The listing builds one solid part. Answer for the finished solid, in the listing's coordinates (mm). A direction names the side the tool comes from. Give positions to 0.01 mm unless a question says otherwise; leave off trailing zeros. Order: outer loops, then holes, each group sorted by start corner. A loop starts at its lowest first (then second) coordinate and runs counter-clockwise, first axis right, second up. Notation, with made-up numbers: (36.5, 51.25) - (61.5, 51.25) arc R3 ccw to (61.5, 55.25) - close; hole circle Ø5 at (50, 63). An arc over 180 degrees is marked (long way). Use CSV: the item, a comma, the result in double quotes.
```python
from build123d import *

# Parameters (mm, degrees)
SKETCH_1_W          = 80
SKETCH_1_H          = 40
EXTRUDE_1_DEPTH     = 9
SKETCH_2_R          = 2.25
CUT_EXTRUDE_1_DEPTH = 46.617978912
SKETCH_3_R          = 2.25
CUT_EXTRUDE_2_DEPTH = 9
SKETCH_4_R          = 4
CUT_EXTRUDE_3_DEPTH = 4.5
SKETCH_6_R          = 4
CUT_EXTRUDE_5_DEPTH = 4.5


with BuildPart() as part:
    # 草图1 → 凸台-拉伸1 (new body)
    with BuildSketch(Plane.XY):
        Rectangle(SKETCH_1_W, SKETCH_1_H)
    extrude(amount=EXTRUDE_1_DEPTH)

    # 草图2 → 切除-拉伸1 (cut, through all)
    with BuildSketch(Plane(origin=(0, 0, 0), x_dir=(-1, 0, 0), z_dir=(0, 0, -1))):
        with Locations((30, 10)):
            Circle(SKETCH_2_R)
        with Locations((30, -10)):
            Circle(SKETCH_2_R)
    cut_extrude_1 = extrude(amount=-CUT_EXTRUDE_1_DEPTH, mode=Mode.SUBTRACT)

    # 镜向1: 切除-拉伸1 across plane
    add(cut_extrude_1.mirror(Plane(origin=(0, 0, 0), x_dir=(0, 0, 1), z_dir=(1, 0, 0))), mode=Mode.SUBTRACT)

    # 草图3 → 切除-拉伸2 (cut)
    with BuildSketch(Plane(origin=(0, 0, 0), x_dir=(-1, 0, 0), z_dir=(0, 0, -1))):
        with Locations((12.5, -12.5)):
            Circle(SKETCH_3_R)
        with Locations((12.5, 12.5)):
            Circle(SKETCH_3_R)
    cut_extrude_2 = extrude(amount=-CUT_EXTRUDE_2_DEPTH, mode=Mode.SUBTRACT)

    # 镜向2: 切除-拉伸2 across plane
    add(cut_extrude_2.mirror(Plane(origin=(0, 0, 0), x_dir=(0, 0, 1), z_dir=(1, 0, 0))), mode=Mode.SUBTRACT)

    # 草图4 → 切除-拉伸3 (cut)
    with BuildSketch(Plane(origin=(0, 0, 0), x_dir=(-1, 0, 0), z_dir=(0, 0, -1))):
        with Locations((12.5, 12.5)):
            Circle(SKETCH_4_R)
        with Locations((12.5, -12.5)):
            Circle(SKETCH_4_R)
        with Locations((-12.5, 12.5)):
            Circle(SKETCH_4_R)
        with Locations((-12.5, -12.5)):
            Circle(SKETCH_4_R)
    extrude(amount=-CUT_EXTRUDE_3_DEPTH, mode=Mode.SUBTRACT)

    # 草图6 → 切除-拉伸5 (cut)
    with BuildSketch(Plane.XY.offset(9)):
        with Locations((-30, -10)):
            Circle(SKETCH_6_R)
        with Locations((-30, 10)):
            Circle(SKETCH_6_R)
        with Locations((30, -10)):
            Circle(SKETCH_6_R)
        with Locations((30, 10)):
            Circle(SKETCH_6_R)
    extrude(amount=-CUT_EXTRUDE_5_DEPTH, mode=Mode.SUBTRACT)


solid = part.part
```
Item 1: The part is cut by section C-C (x = -27). Give the vertices of the cut face in (y, z).
Taken from the geometry:
outline,"(-20, 0) - (20, 0) - (20, 9) - (12.65, 9) - (12.65, 4.5) - (7.35, 4.5) - (7.35, 9) - (-7.35, 9) - (-7.35, 4.5) - (-12.65, 4.5) - (-12.65, 9) - (-20, 9) - close"
Item 2: The mould has two halves that part along Y. Classify faces 1 (the face through (-31.21, -8.103, 2.218)), 2 (the face through (-40, 0, 4)), 3 (the face through (-1, 20, 4)): +Y half, -Y half, draft (parallel to the pull), parting line (faces both ways), or undercut.
Taken from the geometry:
face 1,"undercut"
face 2,"draft"
face 3,"+Y half"
Item 3: Find the intervals of material crossed by line 1 along Y through (x, z) = (30, 7); line 2 along Y through (x, z) = (-12.5, 7.2); line 3 along X through (y, z) = (14.5, 3), in increasing order.
Taken from the geometry:
line 1,"-20 to -14, -6 to 6, 14 to 20"
line 2,"-20 to -14.75, -10.25 to 10.25, 14.75 to 20"
line 3,"-40 to -15.96, -9.04 to 9.04, 15.96 to 40"
Item 4: Each of these flat-tipped pins is pushed along its axis until it touches: pin 1 (6.5 mm diameter, centred on x = -12.5, y = 12.5, fed in from +Z); pin 2 (2.5 mm diameter, centred on x = -31.5, y = -10, fed in from +Z); pin 3 (2.5 mm diameter, centred on x = 13.5, y = 10.5, fed in from -Z). Where does it stop, or does it pass through?
Taken from the geometry:
pin 1,"z = 9"
pin 2,"z = 4.5"
pin 3,"z = 4.5"
Item 5: The part is cut by section B-B (z = 3.25). Count the separate pieces of the cut face and the enclosed holes in it, and give its area (3 significant figures).
Taken from the geometry:
separate pieces,"1"
enclosed holes,"8"
area,"2,940 mm^2"
Item 6: Which of the six approach directions +Z, -Z, +X, -X, +Y, -Y give full straight-line access (tool end or side, diameter ignored) to faces 4 (the face through (-10.84, -10.98, 6.72)), 5 (the face through (15.7, -14.9, 2.2)), 6 (the face through (26, 10, 7))?
Taken from the geometry:
face 4,"+Z, -Z"
face 5,"-Z"
face 6,"+Z"
Item 7: The part is cut by section A-A (x = -12.5). Give the vertices of the cut face in (y, z).
Taken from the geometry:
outline,"(-20, 0) - (-16.5, 0) - (-16.5, 4.5) - (-14.75, 4.5) - (-14.75, 9) - (-20, 9) - close; (-10.25, 4.5) - (-8.5, 4.5) - (-8.5, 0) - (8.5, 0) - (8.5, 4.5) - (10.25, 4.5) - (10.25, 9) - (-10.25, 9) - close; (14.75, 4.5) - (16.5, 4.5) - (16.5, 0) - (20, 0) - (20, 9) - (14.75, 9) - close"
